CAD build for the part. Positions are in the model's coordinates, mm. A direction names the side the tool comes from. Give positions to 0.01 mm unless a question says otherwise; leave off trailing zeros. Order: outer loops, then holes, each group sorted by start corner. A loop starts at its lowest first (then second) coordinate and runs counter-clockwise, first axis right, second up.
Item 1: Band-saw the part on B-B on z = 7. Give the cut face in (x, y).
Item 2: Which spindle directions (+Z, -Z, +X, -X, +Y, -Y) get a long thin tool onto all of the face, cutting with end or side? Do faces 4 (the flat face through (-21.425, 4, 10)), 5 (the flat face through (-8.903, 3, 11)), 6 (the flat face through (21.564, 3, -8)), 7 (the flat face through (25, 3, 6.26)). Say none if no direction does.
Item 3: Band-saw the part on C-C on x = -20. Give the cut face in (y, z) (3 decimals), plus the area to 3 significant figures.
Item 4: Wall check: L1, parallel to X at y = 4.25, z = 14; L2, parallel to Z at x = -8, y = 5; L3, parallel to Z at x = 24, y = 2.25. Give the ranges that are in metal, low to high.
Item 5: Flat gauge pins, fed straight in: P1, Ø3, axis at x = -11.5, y = 4.5, coming from the +Z side; P2, Ø2.5, axis at y = 3, z = -8, coming from the +X side; P3, Ø3, axis at x = 25, y = 2, coming from the +Z side. Where does each tip first touch, or does it go through?
Item 6: Two-plate mould, pull along Z, no slides. Class faces 1 (the flat face through (8.903, 3, 11)), 2 (the flat face through (-25, 3, -6.135)), 3 (the flat face through (-25, 3, 6.26)): released by +Z, released by -Z, zero draft, split by the parting line, or undercut.
Item 7: Band-saw the part on A-A on x = -8. Give the cut face in (y, z), plus the area to 3 significant figures.
```python
from build123d import *

# Parameters (mm, degrees)
BOSS_EXTRUDE1_DEPTH = 6.35
SKETCH3_R           = 1.1303
CUT_EXTRUDE1_DEPTH  = 12.7


with BuildPart() as part:
    # Sketch2 → Boss-Extrude1 (new body)
    with BuildSketch(Plane(origin=(0, 0, 0), x_dir=(1, 0, 0), z_dir=(0, 1, 0))):
        Polygon((-21.4249, -15.91216588), (-6.1976, -15.91216588), (-6.1976, -22.26216588), (6.1976, -22.26216588), (6.1976, -15.91216588), (21.6027, -15.91216588), (21.6027, -6.26016588), (27.914167201, -6.26016588), (27.914167201, 6.13503412), (21.564167201, 6.13503412), (21.564167201, 9.37353412), (-21.463432799, 9.37353412), (-21.463432799, 6.13503412), (-27.813432799, 6.13503412), (-27.813432799, -6.26016588), (-21.4249, -6.26016588), align=None)
    extrude(amount=BOSS_EXTRUDE1_DEPTH)

    # Sketch3 → Cut-Extrude1 (cut)
    with BuildSketch(Plane(origin=(21.6027, 0, 0), x_dir=(0, 0, -1), z_dir=(1, 0, 0))):
        with Locations((-11.08616588, 3.175)):
            Circle(SKETCH3_R)
    cut_extrude1 = extrude(amount=-CUT_EXTRUDE1_DEPTH, mode=Mode.SUBTRACT)

    # Mirror1: Cut-Extrude1 across plane
    add(cut_extrude1.mirror(Plane(origin=(0, 0, 0), x_dir=(0, 0, 1), z_dir=(1, 0, 0))), mode=Mode.SUBTRACT)


solid = part.part
```
The answers:
1. outline: (-21.42, 0) - (21.6, 0) - (21.6, 6.35) - (-21.42, 6.35) - close
2. face 4: +Z, -X, +Y, -Y
2. face 5: -X
2. face 6: -Z, +X, +Y, -Y
2. face 7: +Z, +X, +Y, -Y
3. outline: (0, -9.374) - (6.35, -9.374) - (6.35, 15.912) - (0, 15.912) - close; hole circle Ø2.261 at (3.175, 11.086)
3. area: 157 mm2
4. L1: x = -21.42 to 21.6
4. L2: z = -9.37 to 15.91
4. L3: z = -6.14 to 6.26
5. P1: stops at z = 15.91
5. P2: stops at x = 21.56
5. P3: stops at z = 6.26
6. face 1: undercut
6. face 2: released by -Z
6. face 3: released by +Z
7. outline: (0, -9.37) - (6.35, -9.37) - (6.35, 15.91) - (0, 15.91) - close
7. area: 161 mm2
